```python
from build123d import *

# Parameters (mm, degrees)
SKICA1_R                 = 25
P_IDAT_VYSUNUT_M1_DEPTH  = 26
SKICA2_R                 = 46
P_IDAT_VYSUNUT_M2_DEPTH  = 200
SKICA3_R                 = 25
P_IDAT_VYSUNUT_M3_DEPTH  = 28
SKICA4_R                 = 24.99
P_IDAT_VYSUNUT_M4_DEPTH  = 74
SKICA5_R                 = 12.5
P_IDAT_VYSUNUT_M5_DEPTH  = 28
ZKOSEN_1_SIZE            = 1
ODEBRAT_START            = 12.5
ODEBRAT_VYSUNUT_M2_DEPTH = 4.1
M8_Z_VIT1_D              = 6.8
M8_Z_VIT1_DEPTH          = 25
M8_Z_VIT1_TIP            = 2.042926105


with BuildPart() as part:
    # Skica1 → Přidat vysunutím1 (new body)
    with BuildSketch(Plane.XY):
        with Locations(Location((0, 0, 0), (0, 0, 180))):
            Circle(SKICA1_R)
    extrude(amount=P_IDAT_VYSUNUT_M1_DEPTH)

    # Skica2 → Přidat vysunutím2 (add)
    with BuildSketch(Plane.XY.offset(26)):
        Circle(SKICA2_R)
    extrude(amount=P_IDAT_VYSUNUT_M2_DEPTH)

    # Skica3 → Přidat vysunutím3 (add)
    with BuildSketch(Plane.XY.offset(226)):
        with Locations(Location((0, 0, 0), (0, 0, 180))):
            Circle(SKICA3_R)
    extrude(amount=P_IDAT_VYSUNUT_M3_DEPTH)

    # Skica4 → Přidat vysunutím4 (add)
    with BuildSketch(Plane.XY.offset(254)):
        Circle(SKICA4_R)
    extrude(amount=P_IDAT_VYSUNUT_M4_DEPTH)

    # Skica5 → Přidat vysunutím5 (add)
    with BuildSketch(Plane.XY.offset(328)):
        Circle(SKICA5_R)
    extrude(amount=P_IDAT_VYSUNUT_M5_DEPTH)

    # Zkosení1
    zkosen_1_edges = [part.edges().sort_by_distance(p)[0] for p in [
        (-24.99, 0, 328),
        (25, 0, 0),
        (-12.5, 0, 356),
        (-46, 0, 26),
        (-46, 0, 226),
    ]]
    chamfer(zkosen_1_edges, length=ZKOSEN_1_SIZE)

    # Skica15 → Odebrat rotací12 (revolve, cut)
    with BuildSketch(Plane(origin=(0, 0, 0), x_dir=(0, 0, -1), z_dir=(1, 0, 0)), mode=Mode.PRIVATE) as odebrat_rotac_12_sk:
        with BuildLine():
            Line((-226.4, 24.7), (-227.775735931, 24.7))
            Line((-227.775735931, 24.7), (-228.5, 25))
            Line((-228.5, 25), (-226.012701665, 25))
            ThreePointArc((-226.012701665, 25), (-226.155051026, 24.783772234), (-226.4, 24.7))
        make_face()
        with BuildLine():
            Line((-23.512701665, 25), (-24.28634316, 24.873361621))
            Line((-24.28634316, 24.873361621), (-25.662079091, 24.873361621))
            ThreePointArc((-25.662079091, 24.873361621), (-25.846132218, 24.896407636), (-26, 25))
            Line((-26, 25), (-23.512701665, 25))
        make_face()
        with BuildLine():
            Line((-328, 12.5), (-330.487298335, 12.5))
            Line((-330.487298335, 12.5), (-329.763034266, 12.2))
            Line((-329.763034266, 12.2), (-328.387298335, 12.2))
            ThreePointArc((-328.387298335, 12.2), (-328.14234936, 12.283772234), (-328, 12.5))
        make_face()
    revolve(odebrat_rotac_12_sk.sketch.rotate(Axis((0, 0, 400.442816929), (0, 0, 1)), 90), axis=Axis((0, 0, 400.442816929), (0, 0, 1)), mode=Mode.SUBTRACT)

    # Skica16 → Odebrat vysunutím2 (cut)
    with BuildSketch(Plane(origin=(0, 0, 0), x_dir=(1, 0, 0), z_dir=(0, 1, 0)).offset(ODEBRAT_START)):
        with BuildLine():
            Line((-4, -356), (-4, -332.00000019))
            ThreePointArc((-4, -332.00000019), (0, -328), (4, -332.00000019))
            Line((4, -332.00000019), (4, -356))
            Line((4, -356), (-4, -356))
        make_face()
    extrude(amount=-ODEBRAT_VYSUNUT_M2_DEPTH, mode=Mode.SUBTRACT)

    # Skica17 → Odebrat rotací14 (revolve, cut)
    with BuildSketch(Plane(origin=(0, 0, 0), x_dir=(1, 0, 0), z_dir=(0, 1, 0))):
        Polygon((0, -356), (-7.15, -356), (-5.417949192, -355), (-4.1477786, -352.8), (-4.1477786, -350.5), (-3.4, -349.7522214), (0, -349.7522214), align=None)
    revolve(axis=Axis((0, 0, 356), (0, 0, 1)), mode=Mode.SUBTRACT)

    # M8 závit1
    with Locations(Plane.XY.offset(349.7522214)):
        with Locations((0, 0)):
            Hole(M8_Z_VIT1_D / 2, depth=M8_Z_VIT1_DEPTH)
            with Locations((0, 0, -(M8_Z_VIT1_DEPTH + M8_Z_VIT1_TIP / 2))):  # 118° drill point
                Cone(0, M8_Z_VIT1_D / 2, M8_Z_VIT1_TIP, mode=Mode.SUBTRACT)


solid = part.part
```
The listing builds one solid part. Answer for the finished solid, in the listing's coordinates (mm). A direction names the side the tool comes from. Give positions to 0.01 mm unless a question says otherwise; leave off trailing zeros. Loops run counter-clockwise (first coordinate to the right, second up) from the corner with the lowest first, then second, coordinate; pieces in that order, holes last. Notation, with made-up numbers: (54.5, 23.25) - (96.5, 23.25) arc R19 ccw to (96.5, 37.25) - close; hole circle Ø11 at (-28.75, 15.5). An arc over 180 degrees is marked (long way). Answer as CSV lines item,"result". Start each with the question number.
Item 1: A cutting plane is placed at B-B on z = 309.5. Determine the outline of the cut face in (x, y), then the cut area to 3 significant figures.
Item 2: A cutting plane is placed at A-A on z = 170.5. Determine the outline of the cut face in (x, y), then the cut area to 3 significant figures.
Item 3: For faces 4 (the face through (-23.846, -7.509, 241.072)), 5 (the face through (-5.99, 45.61, 124.61)), 6 (the face through (-23.56, -7.42, 227.1)), determine the directions among +Z, -Z, +X, -X, +Y, -Y from which every point of the face is accessible in a straight line to the end or side of a thin tool.
Item 4: Find the intervals of material crossed by line 1 (X direction, y = 0, z = 351.75); line 2 (X direction, y = 0, z = 343); line 3 (X direction, y = 4, z = 243.5), in increasing order. Write a range as from..to.
Item 5: The mould has two halves that part along X. Classify faces 1 (the face through (19, -19, 226)), 2 (the face through (23.084, -9.571, 289.989)), 3 (the face through (0.74, -3.32, 337.08)): +X half, -X half, draft (parallel to the pull), parting line (faces both ways), or undercut.
Item 6: Each of these flat-tipped pins is pushed along its axis until it touches: pin 1 (5.5 mm diameter, centred on x = 0, y = 0, fed in from +Z); pin 2 (3 mm diameter, centred on y = 9.5, z = 349.5, fed in from +X); pin 3 (4 mm diameter, centred on x = -1, y = 31.5, fed in from -Z). Where does it stop, or does it pass through?
Found:
1,outline,"circle Ø49.98 at (0, 0)"
1,area,"1,960 mm^2"
2,outline,"circle Ø92 at (0, 0)"
2,area,"6,650 mm^2"
3,face 4,"+Z"
3,face 5,"+Z, -Z"
3,face 6,"none"
4,line 1,"x = -12.5..-4.15, 4.15..12.5"
4,line 2,"x = -12.5..-3.4, 3.4..12.5"
4,line 3,"x = -24.68..24.68"
5,face 1,"draft"
5,face 2,"parting line"
5,face 3,"undercut"
6,pin 1,"stops at z = 324.36"
6,pin 2,"stops at x = 9.6"
6,pin 3,"stops at z = 26"
